Geometry: see drawing. Coordinates: mm, zero at the bounding-box minimum. A direction names the side the tool comes from. Round coordinates to 2 decimals unless told otherwise and drop trailing zeros. Loops run counter-clockwise (first coordinate to the right, second up) from the corner with the lowest first, then second, coordinate; pieces in that order, holes last. Notation, with made-up numbers: M 84.25,49.5 L 128.25,49.5 A22 ccw 128.25,84.5 Z; hole C -16,-39.75 d6. An arc over 180 degrees is marked long. Answer as a JSON object with one key per item and string values.
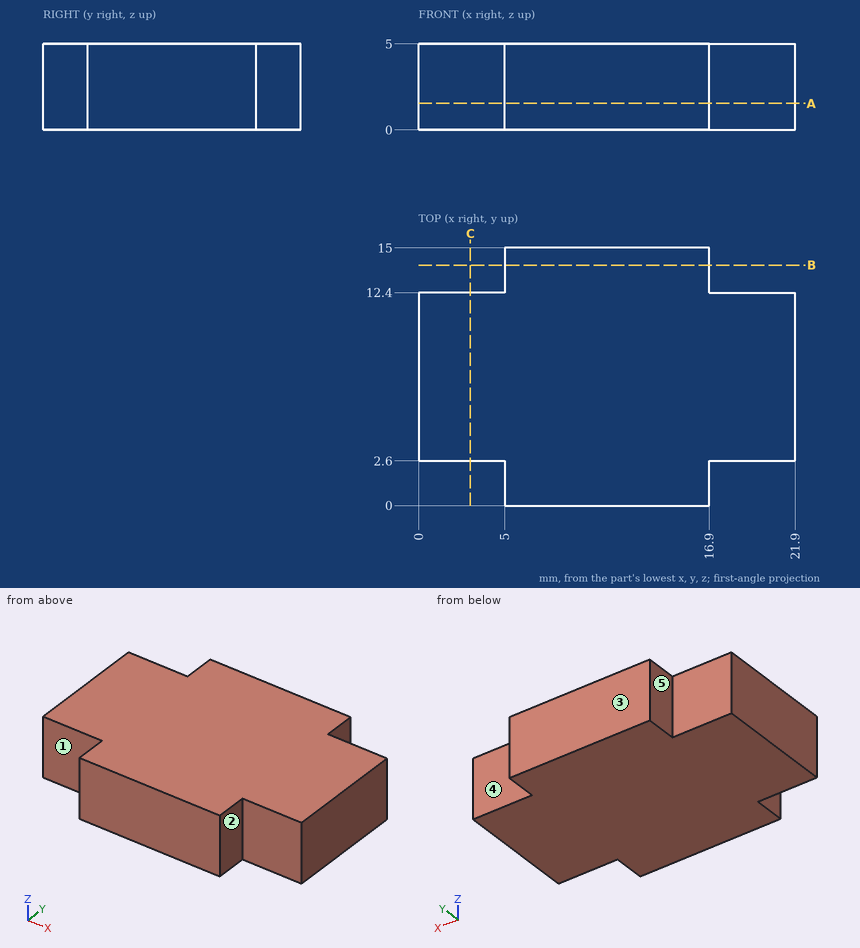
1) Section query A-A (z = 1.55). Return the cut outline in (x, y), and give its area (4 significant figures).
Results:
{"outline": "M 0,2.6 L 5,2.6 L 5,0 L 16.9,0 L 16.9,2.6 L 21.9,2.6 L 21.9,12.4 L 16.9,12.4 L 16.9,15 L 5,15 L 5,12.4 L 0,12.4 Z", "area": "276.5 mm2"}
2) Reachability of the marked faces 1, 2, 3, 4 and 5 from +Z, -Z, +X, -X, +Y, -Y: full face, straight path, thin tool, end or side. Return the list, or none.
Results:
{"face 1": "+Z, -Z, -X, -Y", "face 2": "+Z, -Z, +X, -Y", "face 3": "+Z, -Z, +X, -X, +Y", "face 4": "+Z, -Z, +X, +Y", "face 5": "+Z, -Z, -X, +Y"}
3) Pin query (flat end, axial travel): P1, Ø2.5, axis at x = 19.5, z = 2.5, coming from the +Y side; P2, Ø0.8, axis at y = 14.5, z = 3.5, coming from the +X side; P3, Ø1.3, axis at y = 1.5, z = 1.5, coming from the -X side. Return the tip coordinate at first contact, or that it passes through.
Results:
{"P1": "y = 12.4", "P2": "x = 16.9", "P3": "x = 5"}
4) Section query B-B (y = 14). Return the cut outline in (x, z).
Results:
{"outline": "M 5,0 L 16.9,0 L 16.9,5 L 5,5 Z"}
5) Ray query, line 1 (Y direction, x = 20.5, z = 1.1); line 2 (X direction, y = 13.75, z = 2). Return the intervals inside material, ascending.
Results:
{"line 1": "2.6 to 12.4", "line 2": "5 to 16.9"}
6) Section query C-C (x = 3). Return the cut outline in (y, z), and give its area (3 significant figures).
Results:
{"outline": "M 2.6,0 L 12.4,0 L 12.4,5 L 2.6,5 Z", "area": "49.0 mm2"}
